The listing builds one solid part. Answer for the finished solid, in the listing's coordinates (mm). Face numbers are marked on the shaded views. A direction names the side the tool comes from. Coordinates: 2 decimals unless noted, no trailing zeros. Order: outer loops, then holes, each group sorted by start corner. A loop starts at its lowest first (then second) coordinate and runs counter-clockwise, first axis right, second up. Notation, with made-up numbers: (64, 87.25) -> (94, 87.25) arc R16 cw to (94, 105.25) -> close; hole circle Ø8 at (-37.75, 15.25). An arc over 180 degrees is marked (long way). One line per question, with ' | ' between items.
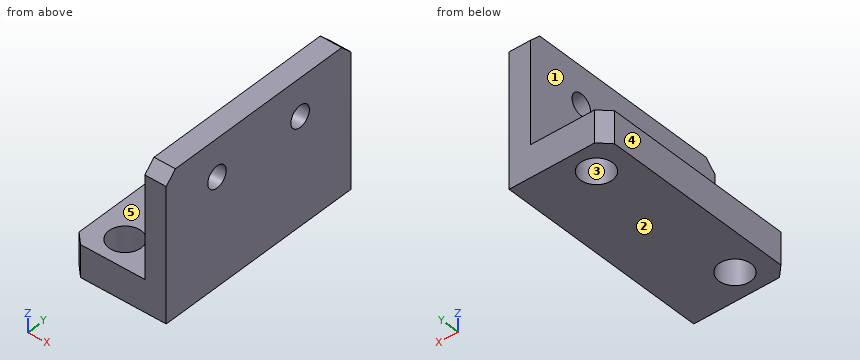
from build123d import *

# Parameters (mm, degrees)
SKETCH_W     = 9
SKETCH_H     = 20
SKETCH_R     = 1.5
PAD_DEPTH    = 3
SKETCH001_W  = 2
SKETCH001_H  = 20
PAD001_DEPTH = 10.5
SKETCH002_R  = 1
POCKET_DEPTH = 5
CHAMFER_SIZE = 1


with BuildPart() as part:
    # Sketch → Pad (new body)
    with BuildSketch(Plane.XY):
        with Locations((4.5, 10)):
            Rectangle(SKETCH_W, SKETCH_H)
        with Locations((3, 17.5)):
            Circle(SKETCH_R, mode=Mode.SUBTRACT)
        with Locations((3, 2.5)):
            Circle(SKETCH_R, mode=Mode.SUBTRACT)
    extrude(amount=PAD_DEPTH)

    # Sketch001 (on Face8 of Pad) → Pad001 (join)
    with BuildSketch(Plane.XY.offset(3)):
        with Locations((8, 10)):
            Rectangle(SKETCH001_W, SKETCH001_H)
    extrude(amount=PAD001_DEPTH)

    # Sketch002 (on Face8 of Pad001) → Pocket (cut)
    with BuildSketch(Plane.YZ.offset(9)):
        with Locations((5.5, 10)):
            Circle(SKETCH002_R)
        with Locations((14.5, 10)):
            Circle(SKETCH002_R)
    extrude(amount=-POCKET_DEPTH, mode=Mode.SUBTRACT)

    # Chamfer
    chamfer_edges = [part.edges().sort_by_distance(p)[0] for p in [
        (8, 0, 13.5),
        (8, 20, 13.5),
        (0, 0, 1.5),
        (0, 20, 1.5),
    ]]
    chamfer(chamfer_edges, length=CHAMFER_SIZE)


solid = part.part
Item 1: Determine the mould class of the marked faces 1, 2 and 3 for opening direction X: pulls with the +X half, pulls with the -X half, needs draft (parallel to the pull), parting line crosses it, or undercut.
Computed values:
face 1: pulls with the -X half | face 2: needs draft | face 3: undercut
Item 2: For the marked faces 4 and 5, determine the directions among +Z, -Z, +X, -X, +Y, -Y from which every point of the face is accessible in a straight line to the end or side of a thin tool.
Computed values:
face 4: +Z, -Z, -X, +Y, -Y | face 5: +Z, -X, +Y, -Y
Item 3: Section D-D, the plane y = 5.5 is taken. Give the vertices of the cut face in (x, z), plus the area to 3 significant figures.
Computed values:
outline: (0, 0) -> (9, 0) -> (9, 9) -> (7, 9) -> (7, 3) -> (0, 3) -> close; (7, 11) -> (9, 11) -> (9, 13.5) -> (7, 13.5) -> close | area: 44.0 mm^2
Item 4: This flat-tipped pin is pushed along its axis until it touches: pin 1 Ø3.5 at (x, y) = (2, 9.5) entering from +Z. Where does it stop, or does it pass through?
Computed values:
pin 1: stops at z = 3
Item 5: Section B-B, the plane z = 10 is taken. Give the vertices of the cut face in (x, y), plus the area to 3 significant figures.
Computed values:
outline: (7, 0) -> (9, 0) -> (9, 4.5) -> (7, 4.5) -> close; (7, 6.5) -> (9, 6.5) -> (9, 13.5) -> (7, 13.5) -> close; (7, 15.5) -> (9, 15.5) -> (9, 20) -> (7, 20) -> close | area: 32.0 mm^2
Item 6: Section A-A, the plane y = 2.5 is taken. Give the vertices of the cut face in (x, z).
Computed values:
outline: (0, 0) -> (1.5, 0) -> (1.5, 3) -> (0, 3) -> close; (4.5, 0) -> (9, 0) -> (9, 13.5) -> (7, 13.5) -> (7, 3) -> (4.5, 3) -> close
Item 7: Find the intervals of material crossed by L1, parallel to Y at x = 3, z = 1.05; L2, parallel to Z at x = 8.3, y = 5.5; L3, parallel to X at y = 13.25, z = 11.75, in increasing order.
Computed values:
L1: y = 0 to 1, 4 to 16, 19 to 20 | L2: z = 0 to 9, 11 to 13.5 | L3: x = 7 to 9
Item 8: Section C-C, the plane x = 3 is taken. Give the vertices of the cut face in (y, z).
Computed values:
outline: (0, 0) -> (1, 0) -> (1, 3) -> (0, 3) -> close; (4, 0) -> (16, 0) -> (16, 3) -> (4, 3) -> close; (19, 0) -> (20, 0) -> (20, 3) -> (19, 3) -> close
